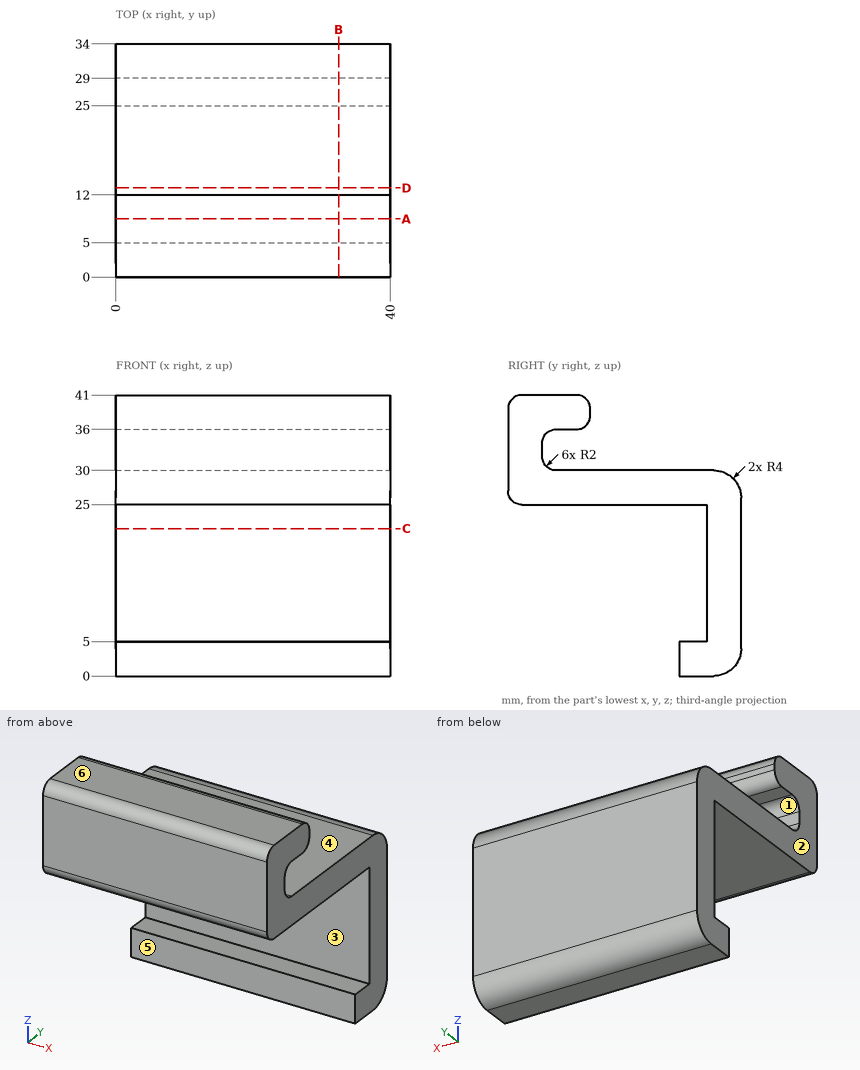
Design review of the part shown in the three views and the two pictorial views. Dimensions are in mm from the part's minimum x, y and z. A direction names the side the tool comes from. Round coordinates to 2 decimals unless told otherwise and drop trailing zeros. Loops run counter-clockwise (first coordinate to the right, second up) from the corner with the lowest first, then second, coordinate; pieces in that order, holes last. Notation, with made-up numbers: M 88,32.5 L 105,32.5 A5 ccw 105,41.5 Z; hole C 67.25,-3.5 d2. An arc over 180 degrees is marked long. Answer as a JSON object with one key per item and string values.
Item 1: Clearance check with flat-ended pins moving along their axes: P1, Ø1.2, axis at x = 27.5, y = 27, coming from the +Z side; P2, Ø6, axis at x = 11.5, z = 17, coming from the -Y side; P3, Ø0.6, axis at x = 13.5, z = 33, coming from the +Y side. State where each tip first meets the part, or that it passes through.
Answer sheet:
{"P1": "stops at z = 30", "P2": "stops at y = 29", "P3": "stops at y = 5"}
Item 2: Machinability: for the marked faces 1, 2 and 3, which of the approach directions +Z, -Z, +X, -X, +Y, -Y give a long, thin tool a straight path to every point of the face, cutting with its end or side? Answer none if there is none.
Answer sheet:
{"face 1": "+X, -X, +Y", "face 2": "+Z, -Z, -X, +Y, -Y", "face 3": "+X, -X, -Y"}
Item 3: We need section B-B on x = 32.5. Give the boundary of the cut face in (y, z), and give its area (3 significant figures).
Answer sheet:
{"outline": "M 0,27 A2 ccw 2,25 L 29,25 L 29,5 L 25,5 L 25,0 L 30,0 A4 ccw 34,4 L 34,26 A4 ccw 30,30 L 7,30 A2 cw 5,32 L 5,34 A2 cw 7,36 L 10,36 A2 ccw 12,38 L 12,39 A2 ccw 10,41 L 2,41 A2 ccw 0,39 Z", "area": "396 mm^2"}
Item 4: The part is to be moulded in two halves that separate along Z. For the marked faces 4, 5 and 6, say which applies: pulls with the +Z half, pulls with the -Z half, needs draft (parallel to the pull), parting line crosses it, or undercut.
Answer sheet:
{"face 4": "undercut", "face 5": "needs draft", "face 6": "pulls with the +Z half"}
Item 5: We need section A-A on y = 8.5. Give the boundary of the cut face in (x, z), and give its area (3 significant figures).
Answer sheet:
{"outline": "M 0,25 L 40,25 L 40,30 L 0,30 Z; M 0,36 L 40,36 L 40,41 L 0,41 Z", "area": "400 mm^2"}
Item 6: Wall thickness on L1, parallel to Z at x = 14, y = 8; L2, parallel to Z at x = 23, y = 26; L3, parallel to Z at x = 16.5, y = 18: over which ranges is each line inside the solid? List them lowest first. Write a range as from..to.
Answer sheet:
{"L1": "z = 25..30, 36..41", "L2": "z = 0..5, 25..30", "L3": "z = 25..30"}
Item 7: We need section D-D on y = 13. Give the boundary of the cut face in (x, z), and give its area (3 significant figures).
Answer sheet:
{"outline": "M 0,25 L 40,25 L 40,30 L 0,30 Z", "area": "200 mm^2"}
Item 8: We need section C-C on z = 21.5. Give the boundary of the cut face in (x, y), and give its area (3 significant figures).
Answer sheet:
{"outline": "M 0,29 L 40,29 L 40,34 L 0,34 Z", "area": "200 mm^2"}
